from build123d import *

# Parameters (mm, degrees)
CHAMFER1_SIZE               = 1.27
F_1_4_20_TAPPED_HOLE1_D     = 5.1054
F_1_4_20_TAPPED_HOLE1_DEPTH = 16.51
F_1_4_20_TAPPED_HOLE1_TIP   = 1.533816902


with BuildPart() as part:
    # Sketch1 → Revolve1 (revolve)
    with BuildSketch(Plane.XY):
        Polygon((0, 0), (12.7, 0), (12.7, 19.05), (9.4996, 19.05), (9.4996, 50.8), (0, 50.8), align=None)
    revolve(axis=Axis((0, 50.8, 0), (0, -1, 0)))

    # Chamfer1
    chamfer1_edges = [part.edges().sort_by_distance(p)[0] for p in [
        (-9.4996, 50.8, 0),
        (-12.7, 0, 0),
    ]]
    chamfer(chamfer1_edges, length=CHAMFER1_SIZE)

    # 1/4-20 Tapped Hole1
    with Locations(Plane(origin=(0, 50.8, 0), x_dir=(1, 0, 0), z_dir=(0, 1, 0))):
        with Locations((0, 0)):
            Hole(F_1_4_20_TAPPED_HOLE1_D / 2, depth=F_1_4_20_TAPPED_HOLE1_DEPTH)
            with Locations((0, 0, -(F_1_4_20_TAPPED_HOLE1_DEPTH + F_1_4_20_TAPPED_HOLE1_TIP / 2))):  # 118° drill point
                Cone(0, F_1_4_20_TAPPED_HOLE1_D / 2, F_1_4_20_TAPPED_HOLE1_TIP, mode=Mode.SUBTRACT)


solid = part.part
The listing builds one solid part. Answer for the finished solid, in the listing's coordinates (mm). Coordinates: 2 decimals unless noted, no trailing zeros. Loops run counter-clockwise (first coordinate to the right, second up) from the corner with the lowest first, then second, coordinate; pieces in that order, holes last. Notation, with made-up numbers: M 72,82 L 108,82 A18 ccw 108,98 Z; hole C 61,65.25 d6. An arc over 180 degrees is marked long. Answer in a Markdown table with one row per item.
1) Given pin 1 (3 mm diameter, centred on x = 5.5, y = 16.5, fed in from -Z); pin 2 (12 mm diameter, centred on x = 0, y = 29, fed in from +Z); pin 3 (4 mm diameter, centred on x = -0.5, y = 45.5, fed in from -Z); pin 4 (2 mm diameter, centred on x = -2.5, z = -4, fed in from -Y), each flat-ended and moving along its own axis, determine where each tip first touches the part or whether it passes through.
Answers below:
| item | result |
|---|---|
| pin 1 | z = -12.05 |
| pin 2 | z = 9.5 |
| pin 3 | z = -9.5 |
| pin 4 | y = 0 |
2) Find section B-B (y = 43). Determine the outline of the cut face in (x, z).
Answers below:
| item | result |
|---|---|
| outline | C 0,0 d19; hole C 0,0 d5.11 |
3) Find section A-A (y = 6.5). Determine the outline of the cut face in (x, z), then the cut area to 3 significant figures.
Answers below:
| item | result |
|---|---|
| outline | C 0,0 d25.4 |
| area | 507 mm^2 |
4) Find section C-C (y = 26). Determine the outline of the cut face in (x, z).
Answers below:
| item | result |
|---|---|
| outline | C 0,0 d19 |
5) Find the intervals of material crossed by probe 1 along Z at (x, y) = (0, 42); probe 2 along Y at (x, z) = (-0.25, 10); probe 3 along X at (y, z) = (36, 0.5), in increasing order.
Answers below:
| item | result |
|---|---|
| probe 1 | -9.5 to -2.55, 2.55 to 9.5 |
| probe 2 | 0 to 19.05 |
| probe 3 | -9.49 to -2.5, 2.5 to 9.49 |
6) Determine the mould class of faces 1 (the flat face through (2.8, 19.05, -9.3)), 2 (the cylindrical face through (-7, 34.5, 6.42)), 3 (the cylindrical face through (-2.435, 42.429, -0.767)) for opening direction Z: released by +Z, released by -Z, zero draft, split by the parting line, or undercut.
Answers below:
| item | result |
|---|---|
| face 1 | zero draft |
| face 2 | split by the parting line |
| face 3 | undercut |
